CAD build for the part. Positions are in the model's coordinates, mm. Face numbers are marked on the shaded views. A direction names the side the tool comes from. Round coordinates to 2 decimals unless told otherwise and drop trailing zeros. Loops run counter-clockwise (first coordinate to the right, second up) from the corner with the lowest first, then second, coordinate; pieces in that order, holes last.
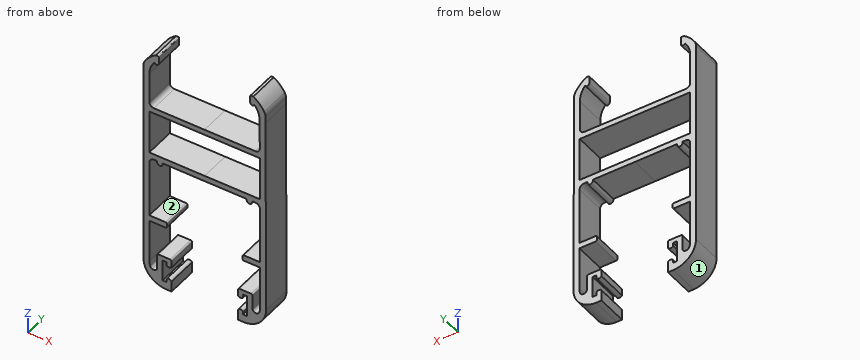
Autodesk Fusion 360 part; units mm, degrees
sketch "Boceto2" plane through (0, 0, 0) normal (0, 1, 0) x (1, 0, 0)
  line L0 (7.5, 0) -> (9.2213, 0)
  line L1 (0, -73.2) -> (0, -7.5)
  arc A0 (7.5, 0) -> (0, -7.5) centre (7.5, -7.5) ccw
  line L2 (7.5, -3.5523) -> (7.5, -2.6)
  line L3 (7.5, -2.6) -> (6.3, -2.6)
  line L4 (6.3, -2.6) -> (6.3, -9.6)
  line L5 (6.3, -9.6) -> (7.5, -9.6)
  line L6 (7.5, -9.6) -> (7.5, -8.5)
  line L7 (9.2213, -8.5) -> (9.2213, -10.6)
  line L8 (8.7213, -11.1) -> (4.9, -11.1)
  line L9 (4.4, -10.6) -> (4.4, -5.7)
  arc A1 (4.4, -5.7) -> (2.8546, -5.0381) centre (3.3076, -6.1153) ccw
  arc A2 (4.4, -5.7) -> (2.1854, -5.7893) centre (3.3076, -6.1153) ccw
  arc A3 (2.1854, -5.7893) -> (1.9172, -7.5) centre (7.5062, -7.5) ccw
  arc A4 (9.2213, -8.5) -> (7.5, -8.5) centre (8.3607, -9.2707) ccw
  arc A5 (7.5, -3.5523) -> (9.2213, -3.5523) centre (8.3607, -3.072) ccw
  line L10 (9.2213, -3.5523) -> (9.2213, 0)
  line L11 (20.1126, -1.9172) -> (20.115, -1.9172)
  line L12 (1.9172, -21.6025) -> (7.2, -21.6025)
  line L13 (7.7, -22.1025) -> (7.7, -23)
  line L14 (7.2, -23.5) -> (1.9172, -23.5)
  line L15 (1.9172, -45.6046) -> (20.0634, -45.6046)
  line L16 (20.0634, -43.7426) -> (20.0634, -43.7426)
  line L17 (20.036, -60.0002) -> (20.036, -60.0234)
  line L18 (20.036, -61.8138) -> (3.4172, -61.8138)
  line L19 (1.9172, -21.6025) -> (1.9172, -7.5)
  arc A6 (7.2, -23.5) -> (7.7, -23) centre (7.2, -23) ccw
  arc A7 (7.7, -22.1025) -> (7.2, -21.6025) centre (7.2, -22.1025) ccw
  line L20 (1.9172, -42.2426) -> (1.9172, -23.5)
  arc A8 (1.9172, -42.2426) -> (3.4172, -43.7426) centre (3.4172, -42.2426) ccw
  line L21 (6.2895, -43.7426) -> (6.2895, -43.415)
  line L22 (4.4317, -43.415) -> (4.4317, -43.7426)
  arc A9 (6.2895, -43.415) -> (4.4317, -43.415) centre (5.3606, -43.415) ccw
  line L23 (20.0634, -43.7426) -> (6.2895, -43.7426)
  line L24 (4.4317, -43.7426) -> (3.4172, -43.7426)
  line L25 (1.9172, -73.2) -> (1.9172, -63.3138)
  line L26 (1.9172, -60.0002) -> (1.9172, -45.6046)
  arc A10 (3.4172, -61.8138) -> (1.9172, -63.3138) centre (3.4172, -63.3138) ccw
  arc A11 (4.4, -10.6) -> (4.9, -11.1) centre (4.9, -10.6) ccw
  arc A12 (8.7213, -11.1) -> (9.2213, -10.6) centre (8.7213, -10.6) ccw
  line L27 (32.4735, -22.1342) -> (32.4712, -23.0317)
  line L28 (35.8029, -10.6401) -> (35.8154, -5.7401)
  arc A13 (36.701, -43.7851) -> (38.2048, -42.289) centre (36.7048, -42.2851) ccw
  line L29 (38.1594, -60.0465) -> (38.1962, -45.651)
  line L30 (33.8286, -43.7778) -> (33.8295, -43.4502)
  arc A14 (35.6873, -43.4549) -> (33.8295, -43.4502) centre (34.7584, -43.4526) ccw
  line L31 (32.7209, -3.5846) -> (32.7233, -2.6322)
  line L32 (35.6864, -43.7825) -> (36.701, -43.7851)
  line L33 (32.9699, -23.5329) -> (38.2527, -23.5464)
  line L34 (40.0429, -73.2512) -> (40.2108, -7.5514)
  line L35 (38.2048, -42.289) -> (38.2527, -23.5464)
  arc A15 (32.4712, -23.0317) -> (32.9699, -23.5329) centre (32.9712, -23.0329) ccw
  line L36 (35.6873, -43.4549) -> (35.6864, -43.7825)
  arc A16 (37.3625, -5.0822) -> (35.8154, -5.7401) centre (36.9067, -6.1583) ccw
  line L37 (30.9869, -8.5278) -> (30.9816, -10.6278)
  arc A17 (38.2936, -7.5465) -> (38.0298, -5.8351) centre (32.7046, -7.5322) ccw
  line L38 (32.73, -0.0322) -> (31.0086, -0.0278)
  arc A18 (40.2108, -7.5514) -> (32.73, -0.0322) centre (32.7108, -7.5322) ccw
  arc A19 (35.3016, -11.1388) -> (35.8029, -10.6401) centre (35.3029, -10.6388) ccw
  arc A20 (32.9748, -21.6355) -> (32.4735, -22.1342) centre (32.9735, -22.1355) ccw
  line L39 (32.7054, -9.6322) -> (32.7082, -8.5322)
  arc A21 (30.9816, -10.6278) -> (31.4803, -11.1291) centre (31.4816, -10.6291) ccw
  line L40 (33.9233, -2.6353) -> (33.9054, -9.6353)
  arc A22 (38.0298, -5.8351) -> (35.8154, -5.7401) centre (36.9067, -6.1583) ccw
  arc A23 (38.151, -63.3601) -> (36.6548, -61.8563) centre (36.651, -63.3563) ccw
  arc A24 (30.9996, -3.5802) -> (32.7209, -3.5846) centre (31.8615, -3.102) ccw
  line L41 (30.9996, -3.5802) -> (31.0086, -0.0278)
  line L42 (38.1257, -73.2463) -> (38.151, -63.3601)
  line L43 (38.2576, -21.649) -> (38.2936, -7.5465)
  line L44 (31.4803, -11.1291) -> (35.3016, -11.1388)
  line L45 (32.7233, -2.6322) -> (33.9233, -2.6353)
  line L46 (33.9054, -9.6353) -> (32.7054, -9.6322)
  arc A25 (32.7082, -8.5322) -> (30.9869, -8.5278) centre (31.8456, -9.3007) ccw
  line L47 (38.2576, -21.649) -> (32.9748, -21.6355)
  line L48 (20.0548, -43.7426) -> (33.8286, -43.7778)
  line L49 (38.1962, -45.651) -> (20.05, -45.6046)
  line L50 (20.036, -61.8138) -> (36.6548, -61.8563)
  line L51 (1.9172, -60.0002) -> (38.1594, -60.0465)
  line L52 (20.036, -61.8138) -> (20.0119, -80.7) construction
  line L53 (20.115, 0) -> (20.0591, -43.7426) construction
  line L54 (20.0567, -45.6046) -> (20.0383, -60.0234) construction
  line L55 (20.0119, -80.7) -> (5.0119, -80.7) construction
  line L56 (5.0119, -80.45) -> (5.0119, -78.1977)
  arc A26 (5.0119, -78.1977) -> (3.6157, -77.9747) centre (4.2942, -78.2091) ccw
  arc A27 (1.9172, -73.2) -> (3.6157, -77.9747) centre (9.4774, -73.2) ccw
  line L57 (4.7619, -80.7) -> (4, -80.7)
  line L58 (0, -73.2) -> (0, -75.4021)
  arc A28 (0.432, -77.0212) -> (4, -80.7) centre (9.4618, -71.8331) ccw
  arc A29 (4.7619, -80.7) -> (5.0119, -80.45) centre (4.7619, -80.45) ccw
  arc A30 (0, -75.4021) -> (0.432, -77.0212) centre (3.25, -75.4021) ccw
  arc A31 (36.415, -78.0166) -> (38.1257, -73.2463) centre (30.5655, -73.2269) ccw
  line L59 (40.0429, -73.2512) -> (40.0372, -75.4532)
  arc A32 (39.6011, -77.0712) -> (40.0372, -75.4532) centre (36.7873, -75.4449) ccw
  arc A33 (36.415, -78.0166) -> (35.0182, -78.2361) centre (35.7359, -78.2493) ccw
  line L60 (35.0125, -80.4883) -> (35.0182, -78.2361)
  arc A34 (35.0125, -80.4883) -> (35.2618, -80.739) centre (35.2625, -80.489) ccw
  arc A35 (36.0237, -80.7409) -> (39.6011, -77.0712) centre (30.5846, -71.8601) ccw
  line L61 (35.2618, -80.739) -> (36.0237, -80.7409)
  point P0 (0, -80.7)
  point P1 (40.2299, -0.0514)
  point P2 (40.2299, -0.0514)
  point P3 (35.0118, -80.7383)
  dimension "d10" = 80.7
  dimension "d14" = 0.5
  dimension "d15" = 1.5
  dimension "d16" = 1.5
  dimension "d17" = 0.5
  dimension "d19" = 15
  dimension "d20" = 0.25
  dimension "d21" = 3.25
extrude "Extruir1" add sketch "Boceto2" along normal blind 10
Item 1: Cut at A-A, the plane x = 27.5. Give the cut face in (y, z).
Answers follow:
outline: (0, 43.76) - (10, 43.76) - (10, 45.62) - (0, 45.62) - close; (0, 60.03) - (10, 60.03) - (10, 61.83) - (0, 61.83) - close
Item 2: 3-axis set-ups, long thin cutter, end or side, ignore diameter. For the marked faces 1 and 2: which of +Z, -Z, +X, -X, +Y, -Y reach the whole face in a straight line?
Answers follow:
face 1: -Z, -X, +Y, -Y
face 2: +Y, -Y
Item 3: Probe line 1 (X direction, y = 3.75, z = 14); line 2 (X direction, y = 0.75, z = 6); line 3 (Z direction, x = 15.5, y = 9). List the from-to ranges inside material, lowest first.
Answers follow:
line 1: x = 0 to 1.92, 38.28 to 40.19
line 2: x = 0.15 to 2.12, 4.4 to 6.3, 33.91 to 35.81, 38.08 to 40.05
line 3: z = 43.74 to 45.6, 60.02 to 61.81
Item 4: Flat gauge pins, fed straight in: P1, Ø0.7, axis at y = 6, z = 79.5, coming from the +X side; P2, Ø6, axis at y = 9, z = 50.5, coming from the +X side; P3, Ø1.1, axis at x = 4, y = 6, coming from the -Z side. Where does each tip first touch, or does it go through?
Answers follow:
P1: stops at x = 38.02
P2: stops at x = 40.11
P3: stops at z = 0.6
Item 5: Cut at B-B, the plane z = 67. Give the cut face in (x, y).
Answers follow:
outline: (0, 0) - (1.92, 0) - (1.92, 10) - (0, 10) - close; (38.14, 0) - (40.06, 0) - (40.06, 10) - (38.14, 10) - close
